Part model, mm, in its own coordinate system. Face numbers are marked on the shaded views. A direction names the side the tool comes from. Coordinates: 2 decimals unless noted, no trailing zeros. Loops run counter-clockwise (first coordinate to the right, second up) from the corner with the lowest first, then second, coordinate; pieces in that order, holes last. Notation, with made-up numbers: (-18, 42) - (-1, 42) arc R19 cw to (-1, 67) - close; hole circle Ø1 at (-12.75, 74). An arc over 180 degrees is marked (long way). Use a Markdown table: item, result. Add a question column.
1. Band-saw the part on C-C, the plane x = 29.5. Give the cut face in (y, z).
2. Band-saw the part on A-A, the plane z = 186.5. Give the cut face in (x, y), plus the area to 3 significant figures.
3. Drop flat-ended pins along their axis: pin 1 (1 mm diameter, centred on x = -134.5, y = 100, fed in from +Z); pin 2 (7 mm diameter, centred on y = 5, z = 3, fed in from -X); pin 3 (7 mm diameter, centred on y = -39, z = 1.5, fed in from +X). Give the stop position or say it passes through.
4. Band-saw the part on B-B, the plane y = -91.5. Give the cut face in (x, z), plus the area to 3 significant figures.
5. Pull direction Y, two halves, no side cores. Call the marked faces 1, 2 and 3: pulls with the +Y half, pulls with the -Y half, needs draft (parallel to the pull), parting line crosses it, or undercut.
6. Wall check: probe 1 along X at (y, z) = (-147, 101); probe 2 along Y at (x, z) = (27, 70); probe 3 along X at (y, z) = (41.5, 94.5). Give the ranges that are in metal, low to high. Write a range as [from, to].
7. 3-axis set-ups, long thin cutter, end or side, ignore diameter. For the marked faces 4, 5 and 6: which of +Z, -Z, +X, -X, +Y, -Y reach the whole face in a straight line?
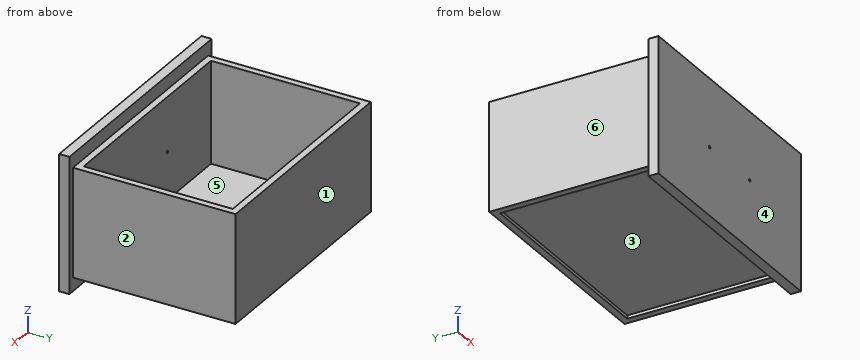
from build123d import *

# Parameters (mm, degrees)
F0_W     = 431.8
F0_H     = 304.8
F0_W_2   = 406.4
F0_H_2   = 279.4
F1_DEPTH = 203.2
F2_W     = 279.4
F2_H     = 6.35
F3_DEPTH = 406.4
F4_W     = 454.152
F4_H     = 254
F5_DEPTH = 19.05
F7_D     = 5.0038
F7_DEPTH = 31.75


with BuildPart() as f1:
    # F0 (on Top) → F1 (new body)
    with BuildSketch(Plane.XY):
        Rectangle(F0_W, F0_H)
        Rectangle(F0_W_2, F0_H_2, mode=Mode.SUBTRACT)
    extrude(amount=F1_DEPTH)

    # F2 (on face) → F3 (join, through all)
    with BuildSketch(Plane.YZ.offset(-203.2)):
        with Locations((0, 9.525)):
            Rectangle(F2_W, F2_H)
    extrude(amount=F3_DEPTH)

    # F4 (on face) → F5 (join)
    with BuildSketch(Plane.XZ.offset(152.4)):
        with Locations((0, 101.6)):
            Rectangle(F4_W, F4_H)
    extrude(amount=F5_DEPTH)

    # F7
    with Locations(Plane.XZ.offset(171.45)):
        with Locations((-64.008, 101.6), (64.008, 101.6)):
            Hole(F7_D / 2, depth=F7_DEPTH)


solid = f1.part
Geometry check:
| question | item | result |
|---|---|---|
| 1 | outline | (-171.45, -25.4) - (-152.4, -25.4) - (-152.4, 0) - (-139.7, 0) - (-139.7, 6.35) - (139.7, 6.35) - (139.7, 0) - (152.4, 0) - (152.4, 203.2) - (139.7, 203.2) - (139.7, 12.7) - (-139.7, 12.7) - (-139.7, 203.2) - (-152.4, 203.2) - (-152.4, 228.6) - (-171.45, 228.6) - close |
| 2 | outline | (-227.08, -171.45) - (227.08, -171.45) - (227.08, -152.4) - (215.9, -152.4) - (215.9, 152.4) - (-215.9, 152.4) - (-215.9, -152.4) - (-227.08, -152.4) - close; hole (-203.2, -139.7) - (203.2, -139.7) - (203.2, 139.7) - (-203.2, 139.7) - close |
| 2 | area | 26,700 mm^2 |
| 3 | pin 1 | stops at z = 12.7 |
| 3 | pin 2 | stops at x = -215.9 |
| 3 | pin 3 | stops at x = 215.9 |
| 4 | outline | (-215.9, 0) - (-203.2, 0) - (-203.2, 6.35) - (203.2, 6.35) - (203.2, 0) - (215.9, 0) - (215.9, 203.2) - (203.2, 203.2) - (203.2, 12.7) - (-203.2, 12.7) - (-203.2, 203.2) - (-215.9, 203.2) - close |
| 4 | area | 7,740 mm^2 |
| 5 | face 1 | pulls with the +Y half |
| 5 | face 2 | needs draft |
| 5 | face 3 | undercut |
| 6 | probe 1 | x = [-215.9, -66.44], [-61.58, 61.58], [66.44, 215.9] |
| 6 | probe 2 | y = [-171.45, -139.7], [139.7, 152.4] |
| 6 | probe 3 | x = [-215.9, -203.2], [203.2, 215.9] |
| 7 | face 4 | +Z, -Z, +X, -X, -Y |
| 7 | face 5 | +Z |
| 7 | face 6 | +Z, -Z, -X, +Y |
